The model under review builds one solid part; all positions refer to its coordinate system, in mm. Face numbers are marked on the shaded views. A direction names the side the tool comes from. Give positions to 0.01 mm unless a question says otherwise; leave off trailing zeros. Loops run counter-clockwise (first coordinate to the right, second up) from the corner with the lowest first, then second, coordinate; pieces in that order, holes last. Notation, with made-up numbers: (25, 52.25) - (74, 52.25) arc R30 ccw to (74, 77.25) - close; hole circle Ø8 at (45.5, -19). An arc over 180 degrees is marked (long way). Return JSON: item names as keys, results as strings. Group by question number.
from build123d import *

# Parameters (mm, degrees)
BOSS_EXTRU_1_DEPTH           = 5
R_P_TITION_CIRCULAIRE1_COUNT = 8
ESQUISSE2_R                  = 5
BOSS_EXTRU_2_DEPTH           = 5


with BuildPart() as part:
    # Esquisse1 → Boss.-Extru.1 (new body)
    with BuildSketch(Plane.XY):
        with BuildLine():
            Line((1.294095226, 4.829629131), (6.470476128, 24.148145657))
            ThreePointArc((6.470476128, 24.148145657), (9.567085809, 23.096988313), (12.5, 21.650635095))
            Line((12.5, 21.650635095), (2.5, 4.330127019))
            ThreePointArc((2.5, 4.330127019), (1.913417162, 4.619397663), (1.294095226, 4.829629131))
        make_face()
    extrude(amount=BOSS_EXTRU_1_DEPTH)


with BuildPart() as r_p_tition_circulaire1_1:
    # R_p_tition circulaire1: pattern copy
    add(part.part.rotate(Axis((0, 0, 0), (0, 0, 1)), 1 * 360 / R_P_TITION_CIRCULAIRE1_COUNT))


with BuildPart() as r_p_tition_circulaire1_2:
    # R_p_tition circulaire1: pattern copy
    add(part.part.rotate(Axis((0, 0, 0), (0, 0, 1)), 2 * 360 / R_P_TITION_CIRCULAIRE1_COUNT))


with BuildPart() as r_p_tition_circulaire1_3:
    # R_p_tition circulaire1: pattern copy
    add(part.part.rotate(Axis((0, 0, 0), (0, 0, 1)), 3 * 360 / R_P_TITION_CIRCULAIRE1_COUNT))


with BuildPart() as r_p_tition_circulaire1_4:
    # R_p_tition circulaire1: pattern copy
    add(part.part.rotate(Axis((0, 0, 0), (0, 0, 1)), 4 * 360 / R_P_TITION_CIRCULAIRE1_COUNT))


with BuildPart() as r_p_tition_circulaire1_5:
    # R_p_tition circulaire1: pattern copy
    add(part.part.rotate(Axis((0, 0, 0), (0, 0, 1)), 5 * 360 / R_P_TITION_CIRCULAIRE1_COUNT))


with BuildPart() as r_p_tition_circulaire1_6:
    # R_p_tition circulaire1: pattern copy
    add(part.part.rotate(Axis((0, 0, 0), (0, 0, 1)), 6 * 360 / R_P_TITION_CIRCULAIRE1_COUNT))


with BuildPart() as r_p_tition_circulaire1_7:
    # R_p_tition circulaire1: pattern copy
    add(part.part.rotate(Axis((0, 0, 0), (0, 0, 1)), 7 * 360 / R_P_TITION_CIRCULAIRE1_COUNT))


with BuildPart() as part_1:
    add(part.part)

    add(r_p_tition_circulaire1_1.part)  # Boss.-Extru.2 merges R_p_tition circulaire1_1

    add(r_p_tition_circulaire1_2.part)  # Boss.-Extru.2 merges R_p_tition circulaire1_2

    add(r_p_tition_circulaire1_3.part)  # Boss.-Extru.2 merges R_p_tition circulaire1_3

    add(r_p_tition_circulaire1_4.part)  # Boss.-Extru.2 merges R_p_tition circulaire1_4

    add(r_p_tition_circulaire1_5.part)  # Boss.-Extru.2 merges R_p_tition circulaire1_5

    add(r_p_tition_circulaire1_6.part)  # Boss.-Extru.2 merges R_p_tition circulaire1_6

    add(r_p_tition_circulaire1_7.part)  # Boss.-Extru.2 merges R_p_tition circulaire1_7
    # Esquisse2 → Boss.-Extru.2 (add)
    with BuildSketch(Plane.XY):
        Circle(ESQUISSE2_R)
    extrude(amount=BOSS_EXTRU_2_DEPTH)


solid = part_1.part
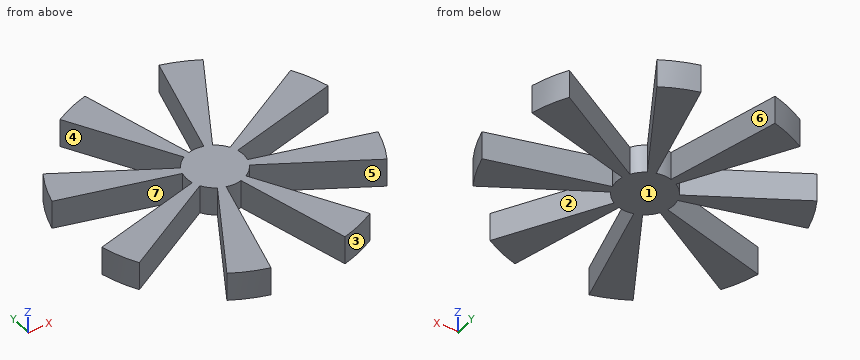
Item 1: For P1, Ø3, axis at x = 9.5, z = 2.5, coming from the -Y side; P2, Ø6, axis at x = -1.5, y = -13, coming from the +Z side; P3, Ø2, axis at y = 15, z = 3, coming from the -X side; P4, Ø1, axis at x = 14.5, z = 1.5, coming from the -Y side, all flat-tipped, find the tip position at first contact; note any pin that passes through.
Item 2: Tool access review of the marked faces 5, 6 and 7: name each direction out of +Z, -Z, +X, -X, +Y, -Y from which nothing blocks a thin tool from reaching the whole face with its end or side.
Item 3: For L1, parallel to X at y = 11, z = 2.6; L2, parallel to Y at x = 9, z = 3.05; L3, parallel to Y at x = 7.5, z = 1, list the stretches that pass through material, from the lowest coordinate up. Write a range as from..to.
Item 4: Mouldability with a two-part tool opening along X and no side actions: class the marked faces 1, 2, 3 and 4 as +X half, -X half, draft (parallel to the pull), parting line (faces both ways), or undercut.
Item 5: Take a section at B-B (y = -21). State the section outline as (x, z) points.
Item 6: Take a section at A-A (x = 16). State the section outline as (y, z) points, then the cut area to 3 significant figures.
Item 7: Take a section at D-D (y = 3.5). State the section outline as (x, z) points.
Check sheet entries:
{
 "1": {"P1": "stops at y = -23.69", "P2": "stops at z = 5", "P3": "stops at x = -9.24", "P4": "stops at y = -8.66"},
 "2": {"face 5": "+Z, -Z", "face 6": "+Z, -Z, +Y", "face 7": "+Z, -Z, -X"},
 "3": {"L1": "x = -22.45..-19.05, -6.35..-2.95, 2.95..6.35, 19.05..22.45", "L2": "y = -23.32..-15.59, -5.2..-2.41, 2.41..5.2, 15.59..23.32", "L3": "y = -23.85..-12.99, -4.33..-2.01, 2.01..4.33, 12.99..23.85"},
 "4": {"face 1": "draft", "face 2": "undercut", "face 3": "+X half", "face 4": "undercut"},
 "5": {"outline": "(-12.12, 0) - (-5.63, 0) - (-5.63, 5) - (-12.12, 5) - close; (5.63, 0) - (12.12, 0) - (12.12, 5) - (5.63, 5) - close"},
 "6": {"outline": "(-9.24, 0) - (-4.29, 0) - (-4.29, 5) - (-9.24, 5) - close; (4.29, 0) - (9.24, 0) - (9.24, 5) - (4.29, 5) - close", "area": "49.5 mm^2"},
 "7": {"outline": "(-13.06, 0) - (-6.06, 0) - (-6.06, 5) - (-13.06, 5) - close; (-3.57, 0) - (3.57, 0) - (3.57, 5) - (-3.57, 5) - close; (6.06, 0) - (13.06, 0) - (13.06, 5) - (6.06, 5) - close"}
}
